Here's the drawing with two shaded views (mm, measured from the low corner). I have some questions. Coordinates: 2 decimals unless noted, no trailing zeros. Order: outer loops, then holes, each group sorted by start corner. A loop starts at its lowest first (then second) coordinate and runs counter-clockwise, first axis right, second up. Notation, with made-up numbers: (-26.75, 13.5) - (-16.75, 13.5) arc R15 cw to (-16.75, 17.5) - close; hole circle Ø9 at (-11, 79.25). An arc over 180 degrees is marked (long way). Answer as CSV lines item,"result". Start each with the question number.
1. I want a section at C-C, the plane x = 6.75. List the corners of the cut face in (y, z) for me (1 decimal).
2. I want a section at A-A, the plane y = 25.4. List the corners of the cut face in (x, z) for me (1 decimal).
3. For pin 1 (7 mm diameter, centred on y = 25.4, z = 6.79, fed in from -X), with a flat end and sliding along its axis, tell me the tip position at first contact or that it passes through.
4. I want a section at B-B, the plane z = 10. List the corners of the cut face in (x, y) for me.
5. I need wall thicknesses on probe 1 along Z at (x, y) = (6.5, 25.4) (1 decimal); probe 2 along Y at (x, z) = (11.5, 8.5) (1 decimal); probe 3 along Y at (x, z) = (3.75, 4.75). Which ranges of each line are inside material? Lowest first, please.
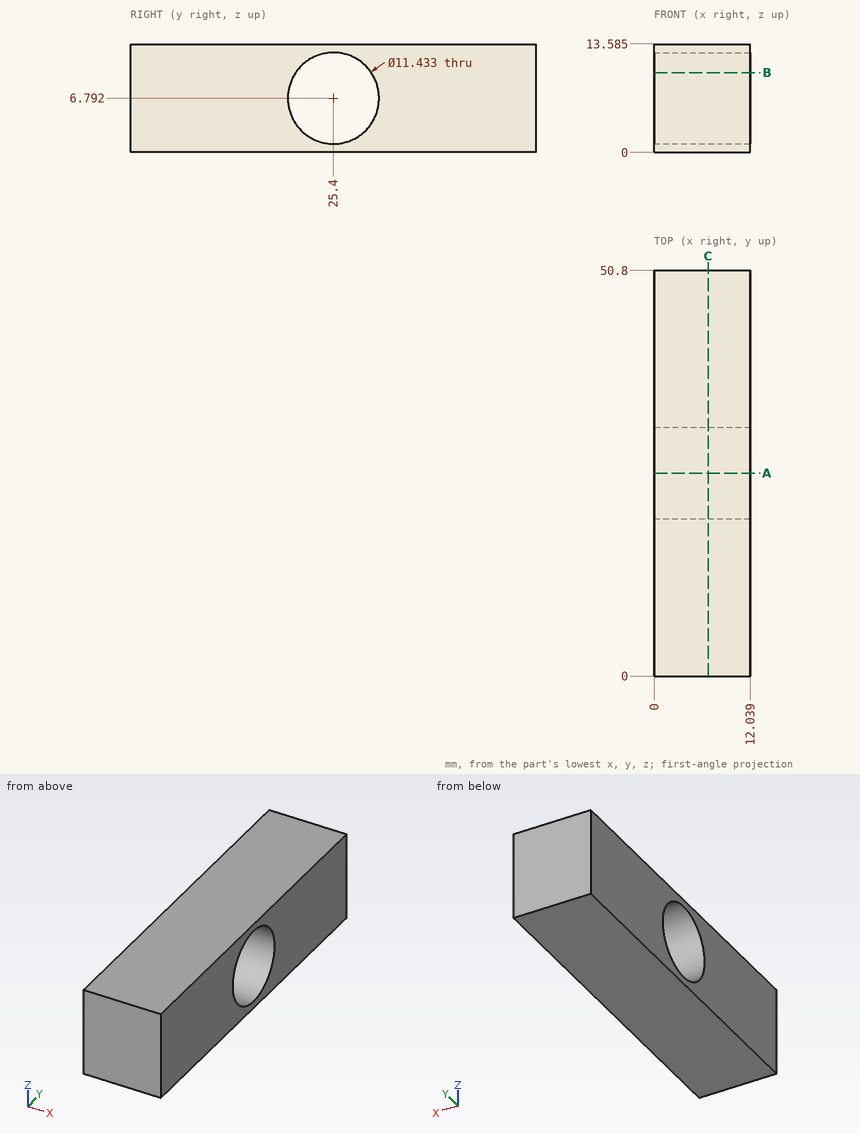
Solved:
1,outline,"(0, 0) - (50.8, 0) - (50.8, 13.6) - (0, 13.6) - close; hole circle Ø11.4 at (25.4, 6.8)"
2,outline,"(0, 0) - (12, 0) - (12, 1.1) - (0, 1.1) - close; (0, 12.5) - (12, 12.5) - (12, 13.6) - (0, 13.6) - close"
3,pin 1,"passes through"
4,outline,"(0, 0) - (12.04, 0) - (12.04, 20.67) - (0, 20.67) - close; (0, 30.13) - (12.04, 30.13) - (12.04, 50.8) - (0, 50.8) - close"
5,probe 1,"z = 0 to 1.1, 12.5 to 13.6"
5,probe 2,"y = 0 to 19.9, 30.9 to 50.8"
5,probe 3,"y = 0 to 20.06, 30.74 to 50.8"
